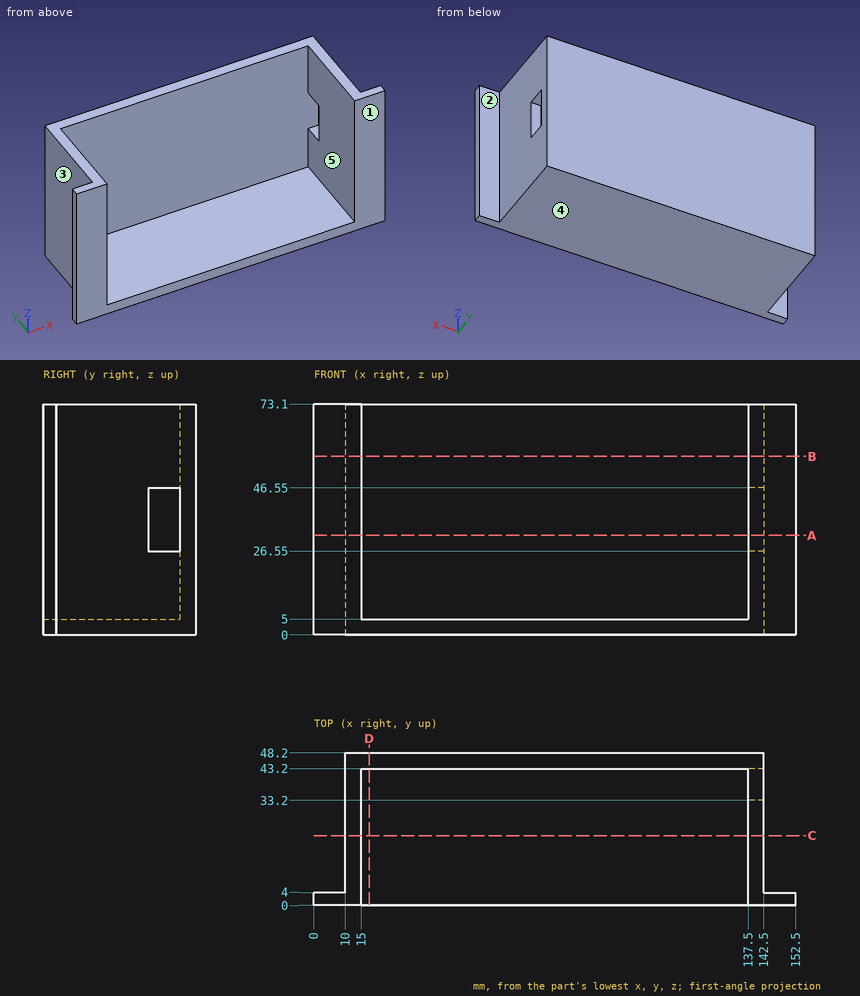
Job drawing, mm, ordinate dimensions from the low corner. One solid piece. A direction names the side the tool comes from. Coordinates: 2 decimals unless noted, no trailing zeros. Write each loop counter-clockwise with the first axis right and the second up, starting at its lowest first coordinate (ties: lowest second). Pieces come first, ordered by that corner, then holes.
Item 1: Slice it at B-B (z = 56.5). Write the cut outline in (x, y).
Item 2: Probe line 1 (X direction, y = 42, z = 48); line 2 (Z direction, x = 67.5, y = 26); line 3 (Y direction, x = 61.5, z = 53). List the from-to ranges inside material, lowest first.
Item 3: Slice it at D-D (x = 17.5). Write the cut outline in (y, z).
Item 4: Slice it at C-C (y = 22). Write the cut outline in (x, z).
Item 5: Pin check, flat tips, straight feed: pin 1 (2 mm diameter, centred on x = 63.5, y = 31.5, fed in from +Z); pin 2 (13 mm diameter, centred on y = 23.5, z = 42.5, fed in from +X); pin 3 (21.5 mm diameter, centred on y = 27, z = 29.5, fed in from -X). Stop position of each tip, or through.
Item 6: Slice it at A-A (z = 31.5). Write the cut outline in (x, y).
Item 7: Which spindle directions (+Z, -Z, +X, -X, +Y, -Y) get a long thin tool onto all of the face, cutting with end or side? Do the marked faces 1, 2, 3, 4 and 5. Say none if no direction does.
Results found:
1. outline: (0, 0) - (15, 0) - (15, 43.2) - (137.5, 43.2) - (137.5, 0) - (152.5, 0) - (152.5, 4) - (142.5, 4) - (142.5, 48.2) - (10, 48.2) - (10, 4) - (0, 4) - close
2. line 1: x = 10 to 15, 137.5 to 142.5
2. line 2: z = 0 to 5
2. line 3: y = 43.2 to 48.2
3. outline: (0, 0) - (48.2, 0) - (48.2, 73.1) - (43.2, 73.1) - (43.2, 5) - (0, 5) - close
4. outline: (10, 0) - (142.5, 0) - (142.5, 73.1) - (137.5, 73.1) - (137.5, 5) - (15, 5) - (15, 73.1) - (10, 73.1) - close
5. pin 1: stops at z = 5
5. pin 2: stops at x = 142.5
5. pin 3: stops at x = 10
6. outline: (0, 0) - (15, 0) - (15, 43.2) - (142.5, 43.2) - (142.5, 48.2) - (10, 48.2) - (10, 4) - (0, 4) - close; (137.5, 0) - (152.5, 0) - (152.5, 4) - (142.5, 4) - (142.5, 33.2) - (137.5, 33.2) - close
7. face 1: +Z, -Z, +X, -X, -Y
7. face 2: +Z, -Z, +X, +Y
7. face 3: +Z, -Z, -X, +Y
7. face 4: -Z, +X, -X, +Y, -Y
7. face 5: +Z, -Y
